Geometry: see drawing. Coordinates: mm, zero at the bounding-box minimum. A direction names the side the tool comes from. Give positions to 0.01 mm unless a question says otherwise; leave off trailing zeros. Loops run counter-clockwise (first coordinate to the right, second up) from the corner with the lowest first, then second, coordinate; pieces in that order, holes last. Notation, with made-up numbers: M -24,-4.75 L 2,-4.75 A16 ccw 2,1.25 Z; hole C -22.5,72.5 d11. An arc over 180 degrees is marked long. Put each result on its own line as item: value.
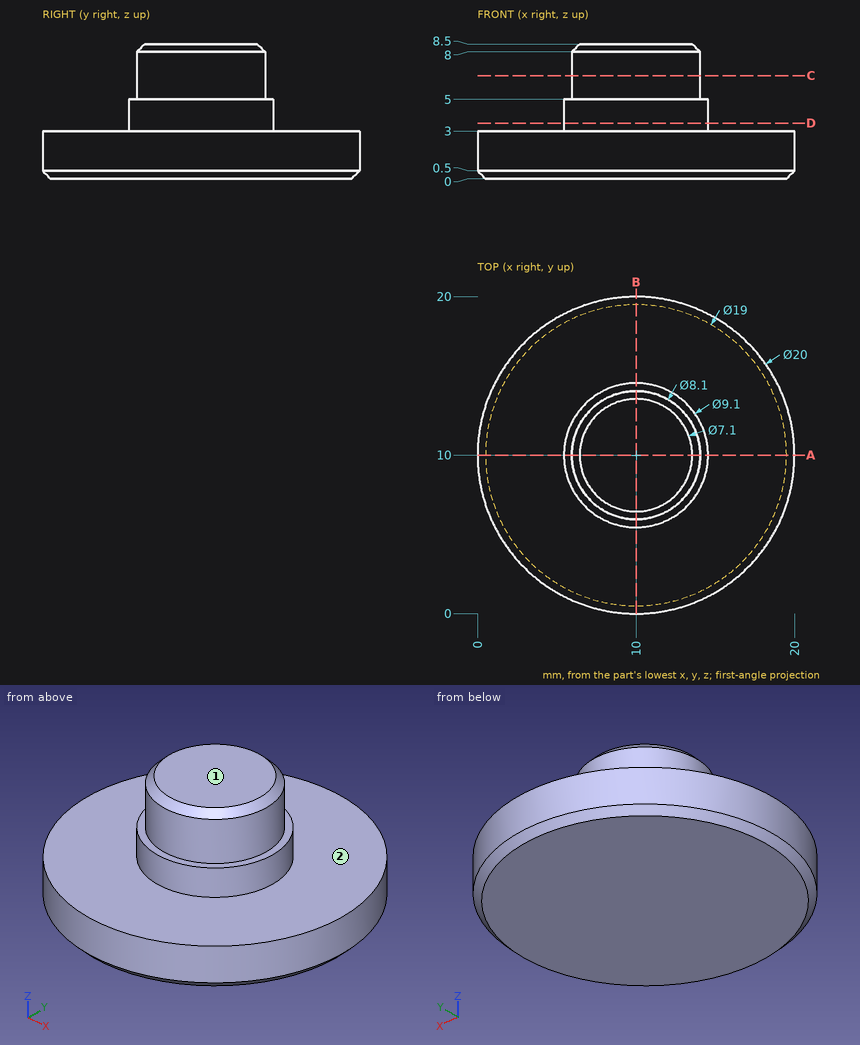
1. Section query D-D (z = 3.5). Output: boundary loops of the cut face in (x, y), plus the area to 3 significant figures.
Found:
outline: C 10,10 d9.1
area: 65.0 mm^2
2. Access query for the marked faces 1 and 2. Directions: +Z, -Z, +X, -X, +Y, -Y. A direction counts if a zero-diameter tool reaches every point of the face in a straight line with its end or side. Return the directions, or none.
Found:
face 1: +Z, +X, -X, +Y, -Y
face 2: +Z
3. Section query C-C (z = 6.5). Output: boundary loops of the cut face in (x, y).
Found:
outline: C 10,10 d8.1
4. Section query A-A (y = 10). Output: boundary loops of the cut face in (x, z), plus the area to 3 significant figures.
Found:
outline: M 0,0.5 L 0.5,0 L 19.5,0 L 20,0.5 L 20,3 L 14.55,3 L 14.55,5 L 14.05,5 L 14.05,8 L 13.55,8.5 L 6.45,8.5 L 5.95,8 L 5.95,5 L 5.45,5 L 5.45,3 L 0,3 Z
area: 106 mm^2
5. Contact query for flat-ended pins moving along their axis: P1, Ø1.5, axis at y = 7, z = 2.5, coming from the +X side; P2, Ø1.5, axis at x = 2.5, z = 1.5, coming from the +Y side. Output: stop coordinate, or through.
Found:
P1: x = 19.74
P2: y = 17.38
6. Material intervals for line 1 (Z direction, x = 6, y = 3); line 2 (Y direction, x = 17.75, z = 1.75); line 3 (Y direction, x = 8, z = 4), sorted ascending. Write a range as from..to.
Found:
line 1: 0..3
line 2: 3.68..16.32
line 3: 5.91..14.09
